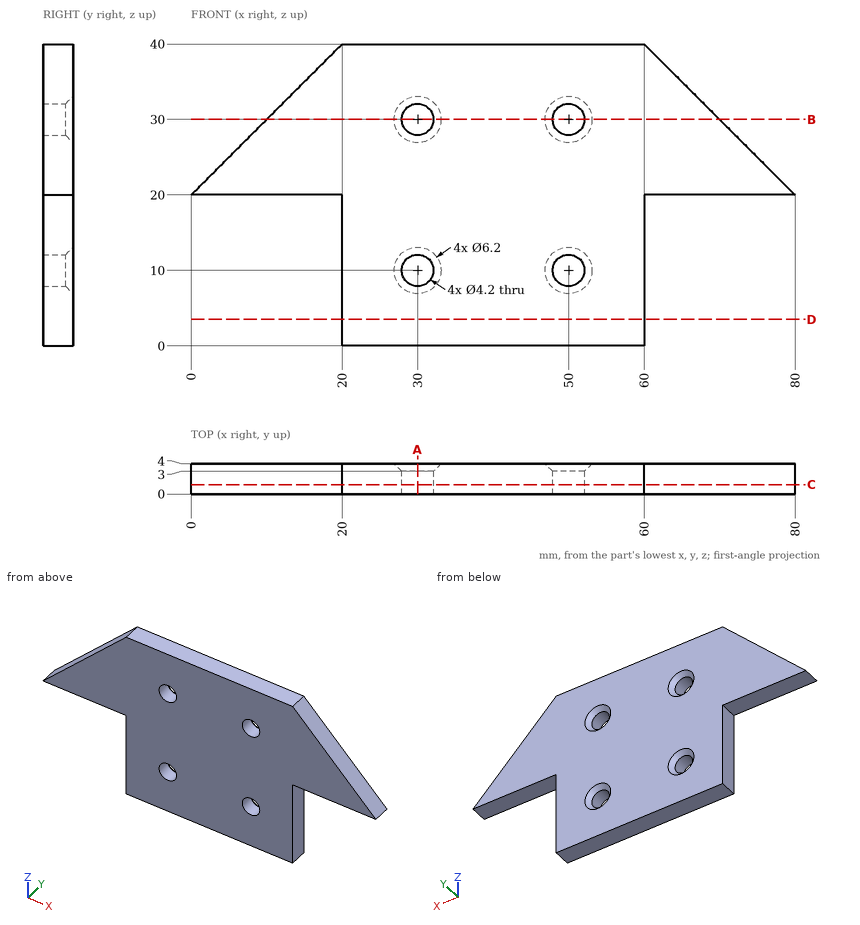
Could you check a few things on this drawing? It's one solid part, dimensions in mm from its lowest x, y, z. Coordinates: 2 decimals unless noted, no trailing zeros. Order: outer loops, then holes, each group sorted by start corner. A loop starts at its lowest first (then second) coordinate and runs counter-clockwise, first axis right, second up.
1. If we section it at D-D (z = 3.5): Please give me the cut outline in (x, y), then the cut area to 3 significant figures.
2. I'm going to push flat-ended pins straight in: pin 1 (1.2 mm diameter, centred on x = 74.5, y = 2, fed in from -Z); pin 2 (2 mm diameter, centred on y = 2, z = 12.5, fed in from -X); pin 3 (6.5 mm diameter, centred on x = 50, z = 10, fed in from +Y); pin 4 (1.5 mm diameter, centred on y = 3.5, z = 23, fed in from -X). Where does each tip first touch, or does it pass through?
3. If we section it at A-A (x = 30): Please give me the cut outline in (y, z).
4. If we section it at C-C (y = 1.25): Please give me the cut outline in (x, z).
5. I need wall thicknesses on line 1 (X direction, y = 2.25, z = 10); line 2 (Z direction, x = 30, y = 1); line 3 (X direction, y = 3.3, z = 10.5). Which ranges of each line are inside material? Lowest first, please.
6. If we section it at B-B (z = 30): Please give me the cut outline in (x, y).
Entries:
1. outline: (20, 0) - (60, 0) - (60, 4) - (20, 4) - close
1. area: 160 mm2
2. pin 1: stops at z = 20
2. pin 2: stops at x = 20
2. pin 3: stops at y = 4
2. pin 4: stops at x = 2.25
3. outline: (0, 0) - (4, 0) - (4, 6.9) - (3, 7.9) - (0, 7.9) - close; (0, 12.1) - (3, 12.1) - (4, 13.1) - (4, 26.9) - (3, 27.9) - (0, 27.9) - close; (0, 32.1) - (3, 32.1) - (4, 33.1) - (4, 40) - (0, 40) - close
4. outline: (0, 20) - (20, 20) - (20, 0) - (60, 0) - (60, 20) - (80, 20) - (60, 40) - (20, 40) - close; hole circle Ø4.2 at (30, 10); hole circle Ø4.2 at (30, 30); hole circle Ø4.2 at (50, 10); hole circle Ø4.2 at (50, 30)
5. line 1: x = 20 to 27.9, 32.1 to 47.9, 52.1 to 60
5. line 2: z = 0 to 7.9, 12.1 to 27.9, 32.1 to 40
5. line 3: x = 20 to 27.65, 32.35 to 47.65, 52.35 to 60
6. outline: (10, 0) - (27.9, 0) - (27.9, 3) - (26.9, 4) - (10, 4) - close; (32.1, 0) - (47.9, 0) - (47.9, 3) - (46.9, 4) - (33.1, 4) - (32.1, 3) - close; (52.1, 0) - (70, 0) - (70, 4) - (53.1, 4) - (52.1, 3) - close
